Geometry: final body of the model. Coordinates: model frame, mm. Face numbers are marked on the shaded views. A direction names the side the tool comes from. Give positions to 0.01 mm unless a question says otherwise; leave off trailing zeros. Loops run counter-clockwise (first coordinate to the right, second up) from the corner with the lowest first, then second, coordinate; pieces in that order, holes last.
from build123d import *

# Parameters (mm, degrees)
OUTPUTSHAFTBASESKETCH_R = 25
PAD005_DEPTH            = 5
HOLESSKETCH_R           = 5.25
POCKET_DEPTH            = 5
PAD006_DEPTH            = 20
DRIVERHOLEPOLAR_COUNT   = 6


with BuildPart() as part:
    # OutputShaftBaseSketch → Pad005 (new body)
    with BuildSketch(Plane.XY):
        Circle(OUTPUTSHAFTBASESKETCH_R)
    extrude(amount=PAD005_DEPTH)

    # holesSketch → Pocket (cut)
    with BuildSketch(Plane.XY):
        with Locations((-19, 0)):
            Circle(HOLESSKETCH_R)
    pocket = extrude(amount=POCKET_DEPTH, mode=Mode.SUBTRACT)

    with BuildSketch(Plane.XY):
        with BuildLine():
            ThreePointArc((-0.979796, 2.3), (0, -2.5), (0.979796, 2.3))
            Line((-0.979796, 2.3), (0.979796, 2.3))
        make_face()
    extrude(amount=PAD006_DEPTH)

    # DriverHolePolar: Pocket ×6 about axis
    driverholepolar_axis = Axis((0, 0, 0), (0, 0, 1))
    for i in range(1, DRIVERHOLEPOLAR_COUNT):
        add(pocket.rotate(driverholepolar_axis, i * 360 / DRIVERHOLEPOLAR_COUNT), mode=Mode.SUBTRACT)


with BuildPart() as part_1:
    # outputShaft placement: moved
    add(part.part.moved(Location((0, 0, 20))))


solid = part_1.part
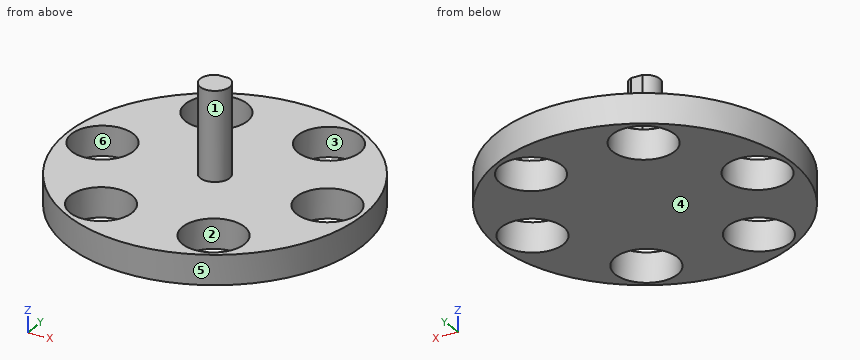
Item 1: Section query C-C on x = 9.5. Return loops of the section in (y, z).
Values follow:
outline: (-23.12, 20) - (-21.7, 20) - (-21.7, 25) - (-23.12, 25) - close; (-11.2, 20) - (11.2, 20) - (11.2, 25) - (-11.2, 25) - close; (21.7, 20) - (23.12, 20) - (23.12, 25) - (21.7, 25) - close
Item 2: Set-up query: the marked faces 1 and 2. Return all of +Z, -Z, +X, -X, +Y, -Y with unobstructed straight access to the full face (end or side cutting, diameter ignored); none if empty.
Values follow:
face 1: +Z
face 2: +Z, -Z
Item 3: Section query A-A on y = 0. Return loops of the section in (x, z).
Values follow:
outline: (-25, 20) - (-24.25, 20) - (-24.25, 25) - (-25, 25) - close; (-13.75, 20) - (13.75, 20) - (13.75, 25) - (2.5, 25) - (2.5, 40) - (-2.5, 40) - (-2.5, 25) - (-13.75, 25) - close; (24.25, 20) - (25, 20) - (25, 25) - (24.25, 25) - close
Item 4: Section query D-D on x = 0. Return loops of the section in (y, z), plus the area to 3 significant figures.
Values follow:
outline: (-25, 20) - (25, 20) - (25, 25) - (2.3, 25) - (2.3, 40) - (-2.5, 40) - (-2.5, 25) - (-25, 25) - close
area: 322 mm2
Item 5: Draft query along X for the marked faces 3, 4, 5 and 6. Return one class per face: +X half, -X half, draft (parallel to the pull), parting line (faces both ways), or undercut.
Values follow:
face 3: undercut
face 4: draft
face 5: parting line
face 6: undercut
Item 6: Ray query, probe 1 along X at (y, z) = (14.5, 24); probe 2 along X at (y, z) = (0.5, 24.5) (3 decimals); probe 3 along Z at (x, y) = (6, 4.5). Return the intervals inside material, ascending.
Values follow:
probe 1: x = -20.37 to -14.37, -4.63 to 4.63, 14.37 to 20.37
probe 2: x = -24.995 to -24.226, -13.774 to 13.774, 24.226 to 24.995
probe 3: z = 20 to 25
Item 7: Pin query (flat end, axial travel): pin 1 (4 mm diameter, centred on x = 5.5, y = -8, fed in from +Z); pin 2 (1 mm diameter, centred on x = 0.5, z = 29.5, fed in from +Y); pin 3 (3 mm diameter, centred on x = -17.5, z = 24, fed in from +Y). Return the tip coordinate at first contact, or that it passes through.
Values follow:
pin 1: stops at z = 25
pin 2: stops at y = 2.3
pin 3: stops at y = 19.21
Item 8: Section query B-B on x = -19. Return loops of the section in (y, z).
Values follow:
outline: (-16.25, 20) - (-5.25, 20) - (-5.25, 25) - (-16.25, 25) - close; (5.25, 20) - (16.25, 20) - (16.25, 25) - (5.25, 25) - close
